Check sheet for the modelled part. Datum: model origin and axes. Units: mm. Give positions to 0.01 mm unless a question says otherwise; leave off trailing zeros. Order: outer loops, then holes, each group sorted by start corner. A loop starts at its lowest first (then second) coordinate and runs counter-clockwise, first axis right, second up. Notation, with made-up numbers: (5.25, -2.5) - (23.25, -2.5) arc R19 ccw to (23.25, 8.5) - close; hole circle Ø1 at (66, -21). An arc over 180 degrees is marked (long way). Answer in a Markdown table with one row per item.
from build123d import *

# Parameters (mm, degrees)
SKETCH1_W           = 1155
SKETCH1_H           = 80
BOSS_EXTRUDE1_DEPTH = 12
SKETCH2_R           = 9
CUT_EXTRUDE1_DEPTH  = 580.007987855
LPATTERN1_COUNT     = 4
LPATTERN1_PITCH     = 366
SKETCH3_W           = 60
SKETCH3_H           = 98
SKETCH3_R           = 10
BOSS_EXTRUDE2_DEPTH = 12


with BuildPart() as part:
    # Sketch1 → Boss-Extrude1 (new body)
    with BuildSketch(Plane(origin=(0, 0, 0), x_dir=(1, 0, 0), z_dir=(0, 1, 0))):
        Rectangle(SKETCH1_W, SKETCH1_H)
    extrude(amount=BOSS_EXTRUDE1_DEPTH)

    # Sketch2 → Cut-Extrude1 (cut, symmetric)
    with BuildSketch(Plane(origin=(0, 12, 0), x_dir=(1, 0, 0), z_dir=(0, 1, 0))):
        with Locations(Location((-549, 0, 0), (0, 0, 270))):
            Circle(SKETCH2_R)
    cut_extrude1 = extrude(amount=CUT_EXTRUDE1_DEPTH, both=True, mode=Mode.SUBTRACT)

    # LPattern1: Cut-Extrude1 ×4
    with Locations(*[(i * LPATTERN1_PITCH, 0, 0) for i in range(1, LPATTERN1_COUNT)]):
        add(cut_extrude1, mode=Mode.SUBTRACT)

    # Sketch3 → Boss-Extrude2 (add)
    with BuildSketch(Plane(origin=(0, 12, 0), x_dir=(1, 0, 0), z_dir=(0, 1, 0))):
        with Locations((-427.5, -89)):
            Rectangle(SKETCH3_W, SKETCH3_H)
        with Locations(Location((-427.5, -108, 0), (0, 0, 270))):
            Circle(SKETCH3_R, mode=Mode.SUBTRACT)
    extrude(amount=-BOSS_EXTRUDE2_DEPTH)


solid = part.part
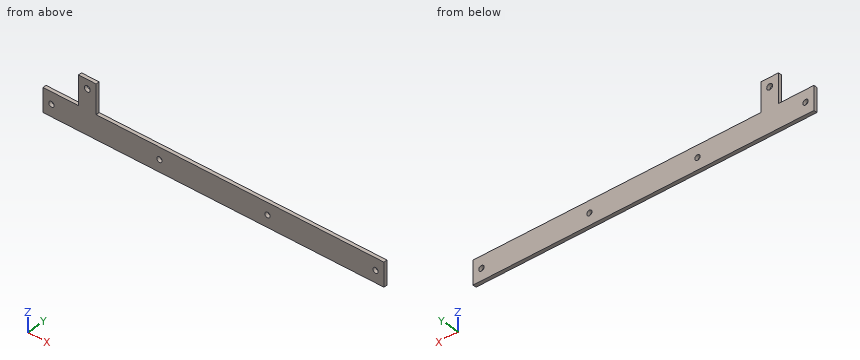
(1) Cross-section at C-C, the plane z = 108. Record the cut outline in (x, y), then the cut area to 3 significant figures.
Geometry says:
| item | result |
|---|---|
| outline | (-457.5, 0) - (-437.5, 0) - (-437.5, 12) - (-457.5, 12) - close; (-417.5, 0) - (-397.5, 0) - (-397.5, 12) - (-417.5, 12) - close |
| area | 480 mm² |
(2) Cross-section at A-A, the plane x = -427.5. Record the cut outline in (y, z).
Geometry says:
| item | result |
|---|---|
| outline | (0, -40) - (12, -40) - (12, 98) - (0, 98) - close; (0, 118) - (12, 118) - (12, 138) - (0, 138) - close |
(3) Cross-section at D-D, the plane x = -164. Record the cut outline in (y, z), then the cut area to 3 significant figures.
Geometry says:
| item | result |
|---|---|
| outline | (0, -40) - (12, -40) - (12, 40) - (0, 40) - close |
| area | 960 mm² |
(4) Thickness scan on L1, parallel to X at y = 2.75, z = 0; L2, parallel to X at y = 4.25, z = -5.5; L3, parallel to X at y = 5.25, z = 41.5. Record the ranges inside material, lowest first.
Geometry says:
| item | result |
|---|---|
| L1 | -577.5 to -558, -540 to -192, -174 to 174, 192 to 540, 558 to 577.5 |
| L2 | -577.5 to -556.12, -541.88 to -190.12, -175.88 to 175.88, 190.12 to 541.88, 556.12 to 577.5 |
| L3 | -457.5 to -397.5 |
(5) Gauge pin test, flat ends, axial feed: P1, Ø18, axis at x = -427.5, z = 108, coming from the +Y side; P2, Ø6, axis at x = -303, y = 7, coming from the +Z side; P3, Ø1.5, axis at y = 10, z = 62, coming from the +X side. Record the tip position at first contact, or that the pin passes through.
Geometry says:
| item | result |
|---|---|
| P1 | through |
| P2 | z = 40 |
| P3 | x = -397.5 |
(6) Cross-section at B-B, the plane y = 4.25. Record the cut outline in (x, z), then the cut area to 3 significant figures.
Geometry says:
| item | result |
|---|---|
| outline | (-577.5, -40) - (577.5, -40) - (577.5, 40) - (-397.5, 40) - (-397.5, 138) - (-457.5, 138) - (-457.5, 40) - (-577.5, 40) - close; hole circle Ø18 at (-549, 0); hole circle Ø20 at (-427.5, 108); hole circle Ø18 at (-183, 0); hole circle Ø18 at (183, 0); hole circle Ø18 at (549, 0) |
| area | 96,900 mm² |
